Part model, mm, in its own coordinate system. A direction names the side the tool comes from. Give positions to 0.01 mm unless a question says otherwise; leave off trailing zeros. Write each loop counter-clockwise with the first axis right and the second up, starting at its lowest first coordinate (ties: lowest second). Pieces come first, ordered by that corner, then holes. Notation, with made-up numbers: (2.25, 44) - (42.25, 44) arc R18 cw to (42.25, 57) - close; hole circle Ø4 at (-8.75, 38). An arc over 180 degrees is marked (long way). Answer as a JSON object with one key per item and string values. Group by question number.
```python
from build123d import *
from build123d import SkipClean  # not in build123d's __all__

# Parameters (mm, degrees)
F1_DEPTH      = 28.575
F2_W          = 76.2
F2_H          = 12.7
F3_DEPTH      = 19.05
F3_DEPTH_BACK = 19.05
F4_R          = 9.525
F5_DEPTH      = 34.926


with BuildPart() as f1:
    # F0 (on Top) → F1 (new body, symmetric)
    with BuildSketch(Plane.XY):
        with BuildLine():
            ThreePointArc((0, 19.05), (-19.05, 0), (0, -19.05))
            Line((0, -19.05), (0, -9.525))
            ThreePointArc((0, -9.525), (-9.525, 0), (0, 9.525))
            Line((0, 9.525), (0, 19.05))
        make_face()
        with BuildLine():
            Line((0, -9.525), (0, -19.05))
            ThreePointArc((0, -19.05), (13.4703841816, -13.4703841816), (19.05, 0))
            ThreePointArc((19.05, 0), (13.4703841816, 13.4703841816), (0, 19.05))
            Line((0, 19.05), (0, 9.525))
            ThreePointArc((0, 9.525), (6.7351920908, 6.7351920908), (9.525, 0))
            ThreePointArc((9.525, 0), (6.7351920908, -6.7351920908), (0, -9.525))
        make_face()
    extrude(amount=F1_DEPTH, both=True)

    # F2 (on Front) → F3 (join, two sides)
    with BuildSketch(Plane.XZ) as f3_sk:
        Rectangle(F2_W, F2_H)
    extrude(amount=-F3_DEPTH)
    extrude(f3_sk.sketch, amount=F3_DEPTH_BACK)

    # F4 (on face) → F5 (cut, through all)
    with BuildSketch(Plane.XY.offset(6.35)):
        Circle(F4_R)
    with SkipClean():  # cleaning this boolean's faces spoils the solid; the shape is the same uncleaned
        extrude(amount=-F5_DEPTH, mode=Mode.SUBTRACT)


solid = f1.part
```
1) Two-plate mould, pull along Y, no slides. Class faces 6 (the flat face through (-38.1, 0, 0)), 7 (the flat face through (-1, -19.05, 0)), 8 (the cylindrical face through (-15.12, -11.59, 17.62)): +Y half, -Y half, draft (parallel to the pull), parting line (faces both ways), or undercut.
2) Saw through at A-A (y = 0). List the corners of the cut face in (x, z) (3 decimals).
3) Saw through at D-D (y = 14). List the corners of the cut face in (x, z) (3 decimals), and give its area (3 significant figures).
4) Drill centre lines: line 1 along Y through (x, z) = (0, -14) (3 decimals); line 2 along Z through (x, y) = (18.5, -10); line 3 along X through (y, z) = (-3, -2). Where is each one in solid material? Low to high. Write a range as from..to.
5) Which spindle directions (+Z, -Z, +X, -X, +Y, -Y) get a long thin tool onto all of the face, cutting with end or side? Do faces 1 (the cylindrical face through (-15.12, -11.59, -17.31)), 2 (the flat face through (27, 0, 6.35)), 3 (the flat face through (27, 0, -6.35)), 4 (the flat face through (-1, 19.05, 0)), 5 (the flat face through (-9, -4, 28.575)). Say none if no direction does.
6) Drop flat-ended pins along their axis: P1, Ø5, axis at x = 23, y = 10, coming from the -Z side; P2, Ø8, axis at y = -11.5, z = -22, coming from the +X side; P3, Ø5, axis at x = 19, z = -16.5, coming from the +Y side. Give the stop position or say it passes through.
7) Saw through at C-C (x = -17). List the corners of the cut face in (y, z) (3 decimals).
8) Saw through at B-B (z = -1.5). List the corners of the cut face in (x, y) (3 decimals), and give its area (3 significant figures).
Checks:
{
 "1": {"face 6": "draft", "face 7": "-Y half", "face 8": "parting line"},
 "2": {"outline": "(-38.1, -6.35) - (-19.05, -6.35) - (-19.05, -28.575) - (-9.525, -28.575) - (-9.525, 28.575) - (-19.05, 28.575) - (-19.05, 6.35) - (-38.1, 6.35) - close; (9.525, -28.575) - (19.05, -28.575) - (19.05, -6.35) - (38.1, -6.35) - (38.1, 6.35) - (19.05, 6.35) - (19.05, 28.575) - (9.525, 28.575) - close"},
 "3": {"outline": "(-38.1, -6.35) - (-12.919, -6.35) - (-12.919, -28.575) - (12.919, -28.575) - (12.919, -6.35) - (38.1, -6.35) - (38.1, 6.35) - (12.919, 6.35) - (12.919, 28.575) - (-12.919, 28.575) - (-12.919, 6.35) - (-38.1, 6.35) - close", "area": "2,120 mm2"},
 "4": {"line 1": "-19.05..-9.525, 9.525..19.05", "line 2": "-6.35..6.35", "line 3": "-38.1..-9.04, 9.04..38.1"},
 "5": {"face 1": "-Z", "face 2": "+Z, +X", "face 3": "-Z, +X", "face 4": "+Z, -Z, +X, -X, +Y", "face 5": "+Z, +X, -X, +Y, -Y"},
 "6": {"P1": "z = -6.35", "P2": "x = 17.51", "P3": "y = 9.52"},
 "7": {"outline": "(-19.05, -6.35) - (-8.597, -6.35) - (-8.597, -28.575) - (8.597, -28.575) - (8.597, -6.35) - (19.05, -6.35) - (19.05, 6.35) - (8.597, 6.35) - (8.597, 28.575) - (-8.597, 28.575) - (-8.597, 6.35) - (-19.05, 6.35) - close"},
 "8": {"outline": "(-38.1, -19.05) - (38.1, -19.05) - (38.1, 19.05) - (-38.1, 19.05) - close; hole circle Ø19.05 at (0, 0)", "area": "2,620 mm2"}
}
